from build123d import *

# Parameters (mm, degrees)
SKETCH015_W     = 60
SKETCH015_H     = 90
PAD007_DEPTH    = 28
FILLET_R        = 20
POCKET008_DEPTH = 87


with BuildPart() as part:
    # Sketch015 (on XY_Plane007 of Origin014) → Pad007 (new body)
    with BuildSketch(Plane.XY):
        with Locations((30, 45)):
            Rectangle(SKETCH015_W, SKETCH015_H)
    extrude(amount=PAD007_DEPTH)

    # Fillet
    fillet_edges = [part.edges().sort_by_distance(p)[0] for p in [
        (0, 45, 0),
        (60, 45, 0),
    ]]
    fillet(fillet_edges, radius=FILLET_R)

    # Sketch017 (on Face8 of Fillet) → Pocket008 (cut)
    with BuildSketch(Plane(origin=(0, 90, 0), x_dir=(-1, 0, 0), z_dir=(0, 1, 0))):
        with BuildLine():
            Line((-58.998235, 25.217793), (-1.00896, 25.217793))
            Line((-1.00896, 25.217793), (-1.00896, 19.810799))
            ThreePointArc((-20, 1.008018), (-6.637701, 6.503914), (-1.00896, 19.810799))
            Line((-20, 1.008018), (-39.561207, 1.008018))
            Line((-39.7511, 1.00322), (-39.561207, 1.008018))
            ThreePointArc((-58.998235, 19.918358), (-53.316531, 6.449738), (-39.7511, 1.00322))
            Line((-58.998235, 25.217793), (-58.998235, 19.918358))
        make_face()
    extrude(amount=-POCKET008_DEPTH, mode=Mode.SUBTRACT)


solid = part.part
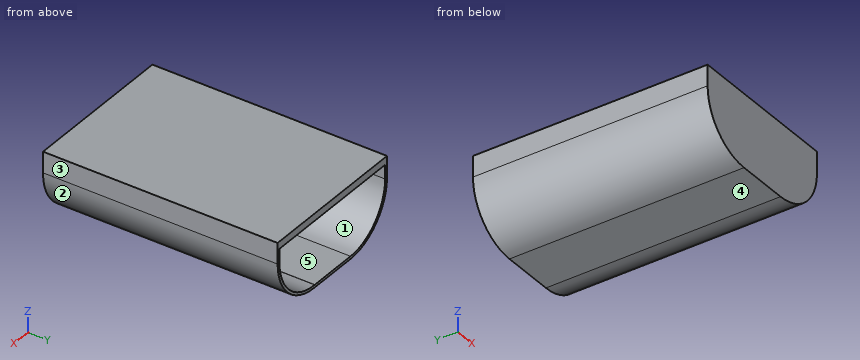
Source: CAD feature listing. Evaluate the final solid. Frame: model axes, mm. Face numbers are marked on the shaded views. A direction names the side the tool comes from. Coordinates: 2 decimals unless noted, no trailing zeros. Order: outer loops, then holes, each group sorted by start corner. A loop starts at its lowest first (then second) coordinate and runs counter-clockwise, first axis right, second up. Notation, with made-up numbers: M 21,25 L 62,25 A22 ccw 62,50 Z; hole C -10.75,-25.5 d3. An arc over 180 degrees is marked long. Write each question's results on one line, items separated by ' | '. Start each with the question number.
Item 1: Cut plane C-C (y = 64). Return loops of the section in (x, z).
Item 2: Line query: probe 1 along Z at (x, y) = (34.5, 35.5); probe 2 along X at (y, z) = (49.5, 24.75); probe 3 along Y at (x, z) = (40.5, 19). Output: solid intervals per line, ascending.
Item 3: Cut plane A-A (z = 23.5). Return loops of the section in (x, y), and give its area (3 significant figures).
Item 4: Cut plane B-B (x = 30). Return loops of the section in (y, z).
Item 5: First-contact query: pin 1 Ø3 at (x, z) = (52, 22.5) entering from -Y; pin 2 Ø2 at (y, z) = (61.5, 4.5) entering from -X (3 decimals); pin 3 Ø6 at (y, z) = (22.5, 14) entering from -X; pin 4 Ø10 at (y, z) = (50, 10.5) entering from +X. Flat tips, straight axial feed; report the tip coordinate or a pass-through.
Item 6: Draft query along X for the marked faces 3, 4 and 5. Return one class per face: pulls with the +X half, pulls with the -X half, needs draft (parallel to the pull), parting line crosses it, or undercut.
Item 7: Set-up query: the marked faces 1 and 2. Return all of +Z, -Z, +X, -X, +Y, -Y with unobstructed straight access to the full face (end or side cutting, diameter ignored); none if empty.
Checked values:
1) outline: M 0,20 A20 ccw 20,0 L 40,0 A20 ccw 60,20 L 60,28 L 0,28 Z; hole M 1.01,19.81 A18.99 ccw 20,1.01 L 39.56,1.01 L 39.75,1 A19 ccw 59,19.92 L 59,25.22 L 1.01,25.22 Z
2) probe 1: z = 0 to 1.01, 25.22 to 28 | probe 2: x = 0 to 1.01, 59 to 60 | probe 3: y = 0 to 3
3) outline: M 0,0 L 60,0 L 60,90 L 59,90 L 59,3 L 1.01,3 L 1.01,90 L 0,90 Z | area: 355 mm2
4) outline: M 0,0 L 90,0 L 90,1.01 L 3,1.01 L 3,25.22 L 90,25.22 L 90,28 L 0,28 Z
5) pin 1: stops at y = 0 | pin 2: stops at x = 6.225 | pin 3: stops at x = 0.23 | pin 4: stops at x = 59.49
6) face 3: pulls with the +X half | face 4: needs draft | face 5: undercut
7) face 1: +Y | face 2: -Z, +X, +Y, -Y
